Read the model definition and answer for the solid it produces. Units are mm, in the model's axes. A direction names the side the tool comes from. Coordinates: 2 decimals unless noted, no trailing zeros. Order: outer loops, then holes, each group sorted by start corner. A loop starts at its lowest first (then second) coordinate and runs counter-clockwise, first axis right, second up. Notation, with made-up numbers: (-14.75, 62) - (33.25, 62) arc R19 ccw to (33.25, 69) - close; hole circle Ø10 at (-31, 57). An arc over 180 degrees is marked (long way). Write item = value, one per line.
from build123d import *

# Parameters (mm, degrees)
SKETCH_R     = 10
PAD_DEPTH    = 3
SKETCH001_R  = 2
PAD001_DEPTH = 5
FILLET_R     = 1
FILLET001_R  = 1


with BuildPart() as part:
    # Sketch → Pad (new body)
    with BuildSketch(Plane.XY):
        Circle(SKETCH_R)
    extrude(amount=PAD_DEPTH)

    # Sketch001 (on Face3 of Pad) → Pad001 (join)
    with BuildSketch(Plane.XY.offset(3)):
        Circle(SKETCH001_R)
    extrude(amount=PAD001_DEPTH)

    # Fillet
    fillet_edges = [part.edges().sort_by_distance(p)[0] for p in [
        (-2, 0, 8),
    ]]
    fillet(fillet_edges, radius=FILLET_R)

    # Fillet001
    fillet001_edges = [part.edges().sort_by_distance(p)[0] for p in [
        (-10, 0, 0),
    ]]
    fillet(fillet001_edges, radius=FILLET001_R)


solid = part.part
1) Straight lines are drawn through the part: line 1 along Z through (x, y) = (3, -7.5); line 2 along Y through (x, z) = (-4, 1.25); line 3 along X through (y, z) = (-8.75, 1.5). For each, find the intervals that lie inside material, in ascending order. Write a range as from..to.
Returned:
line_1 = 0..3
line_2 = -9.17..9.17
line_3 = -4.84..4.84
2) The part is cut by section A-A (z = 1.75). Determine the outline of the cut face in (x, y), and give its area (3 significant figures).
Returned:
outline = circle Ø20 at (0, 0)
area = 314 mm^2
3) Flat-ended cylindrical pins translate along their axes: pin 1 Ø10 at (x, y) = (-3, -0.5) entering from -Z; pin 2 Ø4 at (y, z) = (3, 4) entering from +X; pin 3 Ø1 at (x, y) = (-7, 1.5) entering from +Z. Find the tip coordinate at first contact, or state that the pin passes through.
Returned:
pin_1 = 0
pin_2 = 9.92
pin_3 = 3
4) For faces 1 (the face through (-2.17, -9.76, 1.99)), 2 (the face through (0, -2, 5)), determine the directions among +Z, -Z, +X, -X, +Y, -Y from which every point of the face is accessible in a straight line to the end or side of a thin tool.
Returned:
face_1 = +Z, -Z
face_2 = +Z
5) The part is cut by section B-B (z = 6.75). Determine the outline of the cut face in (x, y).
Returned:
outline = circle Ø4 at (0, 0)
